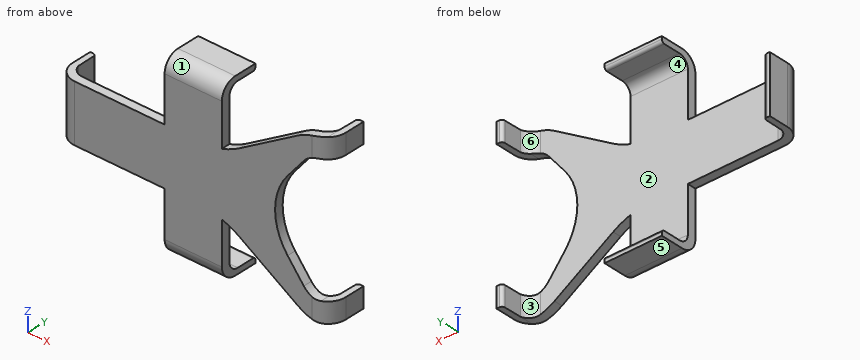
```python
from build123d import *

# Parameters (mm, degrees)
BOSS_EXTRUDE1_DEPTH     = 30
FILLET2_R               = 1
FILLET2_OF_MIRROR4_R    = 1
CUT_EXTRUDE2_DEPTH      = 10.3
CUT_EXTRUDE2_DEPTH_BACK = 3
SKETCH4_OUTSIDE_W       = 120.12
SKETCH4_OUTSIDE_H       = 84.7
BOSS_EXTRUDE2_DEPTH     = 10
FILLET1_R               = 1
FILLET1_OF_MIRROR3_R    = 1


with BuildPart() as part:
    # Sketch3 → Boss-Extrude1 (new, symmetric)
    with BuildSketch(Plane.XY):
        with BuildLine():
            Line((-45.71, 2), (-45.59234107, -4.9990111))
            ThreePointArc((-45.59234107, -4.9990111), (-44.074043193, -7.375333149), (-41.41, -8.3))
            Line((-41.41, -8.3), (0, -8.3))
            Line((0, -8.3), (0, -11.3))
            Line((0, -11.3), (-41.41, -11.3))
            ThreePointArc((-41.41, -11.3), (-45.864772721, -9.454772721), (-47.71, -5))
            Line((-47.71, -5), (-47.71, 2))
            Line((-47.71, 2), (-45.71, 2))
        make_face()
    boss_extrude1 = extrude(amount=BOSS_EXTRUDE1_DEPTH, both=True)

    # Fillet2
    fillet2_edges = [part.edges().sort_by_distance(p)[0] for p in [
        (-45.71, 2, 0),
    ]]
    fillet(fillet2_edges, radius=FILLET2_R)

    # Mirror4: Boss-Extrude1 across plane
    add(boss_extrude1.mirror(Plane(origin=(0, 0, 0), x_dir=(0, 0, 1), z_dir=(1, 0, 0))))

    # Fillet2 of Mirror4
    fillet2_of_mirror4_edges = [part.edges().sort_by_distance(p)[0] for p in [
        (45.71, 2, 0),
    ]]
    fillet(fillet2_of_mirror4_edges, radius=FILLET2_OF_MIRROR4_R)

    # Sketch4 outside → Cut-Extrude2 (cut, two sides: drawn at the far end of the back side and taken through both)
    with BuildSketch(Plane(origin=(0, -8.3, 0), x_dir=(1, 0, 0), z_dir=(0, 1, 0)).offset(-CUT_EXTRUDE2_DEPTH_BACK)):
        Rectangle(SKETCH4_OUTSIDE_W, SKETCH4_OUTSIDE_H)
        with BuildLine():
            Line((-47.71, 10), (2.828114646, 10))
            ThreePointArc((2.828114646, 10), (9.721935767, 10.969285688), (16.081190316, 13.801981572))
            Line((16.081190316, 13.801981572), (36.574790585, 26.614652531))
            ThreePointArc((36.574790585, 26.614652531), (40.899083679, 28.540885732), (45.586882041, 29.2))
            Line((45.586882041, 29.2), (47.71, 29.2))
            Line((47.71, 29.2), (47.71, 22.2))
            Line((47.71, 22.2), (44.078732881, 22.2))
            ThreePointArc((44.078732881, 22.2), (41.043221434, 21.507588307), (38.608231021, 19.567334358))
            Line((38.608231021, 19.567334358), (32.948592182, 12.478098166))
            ThreePointArc((32.948592182, 12.478098166), (28.578597498, 0), (32.948592182, -12.478098166))
            Line((32.948592182, -12.478098166), (38.608231021, -19.567334358))
            ThreePointArc((38.608231021, -19.567334358), (41.043221434, -21.507588307), (44.078732881, -22.2))
            Line((44.078732881, -22.2), (47.71, -22.2))
            Line((47.71, -22.2), (47.71, -29.2))
            Line((47.71, -29.2), (45.586882041, -29.2))
            ThreePointArc((45.586882041, -29.2), (40.899083679, -28.540885732), (36.574790585, -26.614652531))
            Line((36.574790585, -26.614652531), (16.081190316, -13.801981572))
            ThreePointArc((16.081190316, -13.801981572), (9.721935767, -10.969285688), (2.828114646, -10))
            Line((2.828114646, -10), (-47.71, -10))
            Line((-47.71, -10), (-47.71, 10))
        make_face(mode=Mode.SUBTRACT)
    extrude(amount=CUT_EXTRUDE2_DEPTH + CUT_EXTRUDE2_DEPTH_BACK, mode=Mode.SUBTRACT)

    # Sketch2 → Boss-Extrude2 (add, symmetric)
    with BuildSketch(Plane(origin=(0, 0, 0), x_dir=(0, 0, -1), z_dir=(1, 0, 0))):
        with BuildLine():
            Line((-29.2, 2), (-29.2, -5))
            ThreePointArc((-29.2, -5), (-28.233452378, -7.333452378), (-25.9, -8.3))
            Line((-25.9, -8.3), (0, -8.3))
            Line((0, -8.3), (0, -11.3))
            Line((0, -11.3), (-25.9, -11.3))
            ThreePointArc((-25.9, -11.3), (-29.64766594, -9.74766594), (-31.2, -6))
            Line((-31.2, -6), (-31.2, 2))
            Line((-31.2, 2), (-29.2, 2))
        make_face()
    boss_extrude2 = extrude(amount=BOSS_EXTRUDE2_DEPTH, both=True)

    # Fillet1
    fillet1_edges = [part.edges().sort_by_distance(p)[0] for p in [
        (0, 2, 29.2),
    ]]
    fillet(fillet1_edges, radius=FILLET1_R)

    # Mirror3: Boss-Extrude2 across plane
    add(boss_extrude2.mirror(Plane.XY))

    # Fillet1 of Mirror3
    fillet1_of_mirror3_edges = [part.edges().sort_by_distance(p)[0] for p in [
        (0, 2, -29.2),
    ]]
    fillet(fillet1_of_mirror3_edges, radius=FILLET1_OF_MIRROR3_R)


solid = part.part
```
Check sheet for the modelled part. Datum: model origin and axes. Units: mm. Face numbers are marked on the shaded views. A direction names the side the tool comes from. Coordinates: 2 decimals unless noted, no trailing zeros. Loops run counter-clockwise (first coordinate to the right, second up) from the corner with the lowest first, then second, coordinate; pieces in that order, holes last.
1) Material ranges on probe 1 along Y at (x, z) = (8, -7); probe 2 along X at (y, z) = (-5, 0.5); probe 3 along Z at (x, y) = (35, -9.5), recorded low to high.
2) Sectioned sample at A-A (y = -0.75). Record the boundary of the cut face in (x, z).
3) Sectioned sample at D-D (z = 2). Record the boundary of the cut face in (x, y), and give its area (3 significant figures).
4) Gauge pin test, flat ends, axial feed: pin 1 (4 mm diameter, centred on x = 45.5, y = -5, fed in from +Z); pin 2 (3 mm diameter, centred on x = -16, z = -7.5, fed in from +Y); pin 3 (1.1 mm diameter, centred on x = 46.5, y = -6.5, fed in from -Z). Record the tip position at first contact, or that the pin passes through.
5) Release check for a two-part mould opening along Z. For the marked faces 4, 5 and 6 record: released by +Z, released by -Z, zero draft, split by the parting line, or undercut.
6) Sectioned sample at C-C (x = -7.5). Record the boundary of the cut face in (y, z).
7) Access from +Z, -Z, +X, -X, +Y, -Y to the whole of each face (thin tool, end or side, straight path). Record for the marked faces 1, 2 and 3.
8) Sectioned sample at B-B (z = -17.5). Record the boundary of the cut face in (x, y), and give its area (3 significant figures).
Check sheet entries:
1. probe 1: y = -11.3 to -8.3
1. probe 2: x = -47.71 to -45.59
1. probe 3: z = -25.63 to -15.05, 15.05 to 25.63
2. outline: (-47.71, -10) - (-45.66, -10) - (-45.66, 10) - (-47.71, 10) - close; (-10, -31.2) - (10, -31.2) - (10, -29.2) - (-10, -29.2) - close; (-10, 29.2) - (10, 29.2) - (10, 31.2) - (-10, 31.2) - close; (45.66, -29.2) - (47.71, -29.2) - (47.71, -22.2) - (45.66, -22.2) - close; (45.66, 22.2) - (47.71, 22.2) - (47.71, 29.2) - (45.66, 29.2) - close
3. outline: (-47.71, -5) arc R6.3 ccw to (-41.41, -11.3) - (28.68, -11.3) - (28.68, -8.3) - (-41.41, -8.3) arc R4.3 cw to (-45.59, -5) - (-45.69, 1.02) arc R1 ccw to (-46.69, 2) - (-47.71, 2) - close
3. area: 245 mm2
4. pin 1: stops at z = 29.2
4. pin 2: stops at y = -8.3
4. pin 3: stops at z = -29.2
5. face 4: undercut
5. face 5: released by -Z
5. face 6: zero draft
6. outline: (-11.3, -25.9) arc R5.3 ccw to (-6, -31.2) - (2, -31.2) - (2, -30.2) arc R1 ccw to (1, -29.2) - (-5, -29.2) arc R3.3 cw to (-8.3, -25.9) - (-8.3, 25.9) arc R3.3 cw to (-5, 29.2) - (1, 29.2) arc R1 ccw to (2, 30.2) - (2, 31.2) - (-6, 31.2) arc R5.3 ccw to (-11.3, 25.9) - close
7. face 1: +Z, -X, -Y
7. face 2: +Y
7. face 3: +Z, -Z, +Y
8. outline: (-10, -11.3) - (10, -11.3) - (10, -8.3) - (-10, -8.3) - close; (22, -11.3) - (36.96, -11.3) - (36.96, -8.3) - (22, -8.3) - close
8. area: 105 mm2
